The listing builds one solid part. Answer for the finished solid, in the listing's coordinates (mm). Coordinates: 2 decimals unless noted, no trailing zeros. Write each loop counter-clockwise with the first axis right and the second up, starting at its lowest first coordinate (ties: lowest second). Pieces come first, ordered by that corner, then holes.
```python
from build123d import *

# Parameters (mm, degrees)
EXTRUDE_1_DEPTH     = 6
FILLET_1_R          = 1
SKETCH_2_R          = 6.5
CUT_EXTRUDE_1_DEPTH = 179.931854445
FILLET_2_R          = 5


with BuildPart() as part:
    # 草图1 → 凸台-拉伸1 (new body)
    with BuildSketch(Plane(origin=(0, 0, 0), x_dir=(1, 0, 0), z_dir=(0, 1, 0))):
        with BuildLine():
            Line((-11.483876828, 51.544081798), (18.516123172, 51.544081798))
            ThreePointArc((18.516123172, 51.544081798), (36.193792702, 44.221751328), (43.516123172, 26.544081798))
            Line((43.516123172, 26.544081798), (43.516123172, -148.455918202))
            ThreePointArc((43.516123172, -148.455918202), (36.193792702, -166.133587732), (18.516123172, -173.455918202))
            Line((18.516123172, -173.455918202), (-11.483876828, -173.455918202))
            ThreePointArc((-11.483876828, -173.455918202), (-29.161546358, -166.133587732), (-36.483876828, -148.455918202))
            Line((-36.483876828, -148.455918202), (-36.483876828, 26.544081798))
            ThreePointArc((-36.483876828, 26.544081798), (-29.161546358, 44.221751328), (-11.483876828, 51.544081798))
        make_face()
    extrude(amount=EXTRUDE_1_DEPTH)

    # 圆角1
    fillet_1_edges = [part.edges().sort_by_distance(p)[0] for p in [
        (36.193792702, 6, -44.221751328),
        (3.516123172, 6, -51.544081798),
        (-29.161546358, 6, -44.221751328),
        (-36.483876828, 6, 60.955918202),
        (-29.161546358, 6, 166.133587732),
        (3.516123172, 6, 173.455918202),
        (36.193792702, 6, 166.133587732),
        (43.516123172, 6, 60.955918202),
    ]]
    fillet(fillet_1_edges, radius=FILLET_1_R)

    # 草图2 → 切除-拉伸1 (cut, through all)
    with BuildSketch(Plane(origin=(0, 6, 0), x_dir=(1, 0, 0), z_dir=(0, 1, 0))):
        with Locations(Location((3.516123172, 0, 0), (0, 0, 270))):
            Circle(SKETCH_2_R)
    extrude(amount=-CUT_EXTRUDE_1_DEPTH, mode=Mode.SUBTRACT)

    # 圆角2
    fillet_2_edges = [part.edges().sort_by_distance(p)[0] for p in [
        (3.516123172, 6, -6.5),
    ]]
    fillet(fillet_2_edges, radius=FILLET_2_R)


solid = part.part
```
(1) Find the intervals of material crossed by probe 1 along X at (y, z) = (0.6, 0); probe 2 along Z at (x, y) = (-12, 3.5); probe 3 along Z at (x, y) = (1, 0.75), in increasing order.
(2) Section A-A, the plane z = 0 is taken. Write down the section's boundary in (x, y), plus the area to 3 significant figures.
(3) For a pull along X with two mould halves and no side action, classify faces 1 (the cylindrical face through (7.9, 0.5, -4.8)), 2 (the flat face through (43.516, 2, 60)), 3 (the flat face through (4, 6, 59)) as pulls with the +X half, pulls with the -X half, needs draft (parallel to the pull), parting line crosses it, or undercut.
(4) Section B-B, the plane y = 2.5 is taken. Write down the section's boundary in (x, z), plus the area to 3 significant figures.
(5) This flat-tipped pin is pushed along its axis until it touches: pin 1 (8 mm diameter, centred on x = 3.52, z = 0, fed in from -Y). Where does it stop, or does it pass through?
Solution:
1. probe 1: x = -36.48 to -2.98, 10.02 to 43.52
1. probe 2: z = -51.54 to 173.45
1. probe 3: z = -51.54 to -5.99, 5.99 to 173.46
2. outline: (-36.48, 0) - (-2.98, 0) - (-2.98, 1) arc R5 ccw to (-7.98, 6) - (-35.48, 6) arc R1 ccw to (-36.48, 5) - close; (10.02, 0) - (43.52, 0) - (43.52, 5) arc R1 ccw to (42.52, 6) - (15.02, 6) arc R5 ccw to (10.02, 1) - close
2. area: 391 mm2
3. face 1: undercut
3. face 2: pulls with the +X half
3. face 3: needs draft
4. outline: (-36.48, -26.54) arc R25 ccw to (-11.48, -51.54) - (18.52, -51.54) arc R25 ccw to (43.52, -26.54) - (43.52, 148.46) arc R25 ccw to (18.52, 173.46) - (-11.48, 173.46) arc R25 ccw to (-36.48, 148.46) - close; hole circle Ø13.46 at (3.52, 0)
4. area: 17,300 mm2
5. pin 1: passes through
